Geometry check sheet. Reference: the model listing, model coordinates, mm. Face numbers are marked on the shaded views. A direction names the side the tool comes from. Give positions to 0.01 mm unless a question says otherwise; leave off trailing zeros. Write each loop counter-clockwise with the first axis right and the second up, starting at its lowest first coordinate (ties: lowest second). Pieces come first, ordered by that corner, then holes. Notation, with made-up numbers: (51, -1.75) - (90, -1.75) arc R20 ccw to (90, 24.25) - close; hole circle Ø7 at (31.5, -28.75). An arc over 180 degrees is marked (long way). Use a Markdown table: item, result.
```python
from build123d import *

# Parameters (mm, degrees)
SKETCH1_W          = 140
SKETCH1_H          = 8.92
BASE_FLANGE1_DEPTH = 2.5
EDGE_FLANGE1_DEPTH = 140
SKETCH21_R         = 1.65
CUT_EXTRUDE1_DEPTH = 78.265670645
CHAMFER1_SIZE      = 3
CHAMFER1_SIZE2     = 24.433039284
FILLET1_R          = 0.5


# Sheet-metal steps are written as plain solids
with BuildPart() as part:
    # Sketch1 → Base-Flange1 (new body)
    with BuildSketch(Plane(origin=(0, 0, 0), x_dir=(1, 0, 0), z_dir=(0, 1, 0))):
        with Locations((0, -4.46)):
            Rectangle(SKETCH1_W, SKETCH1_H)
    extrude(amount=-BASE_FLANGE1_DEPTH)

    # Edge-Flange1 section (across the edge) → Edge-Flange1 (add)
    with BuildSketch(Plane(origin=(70, -2.5, 9.759099631), x_dir=(0, -0.17364817766693427, -0.9848077530122075), z_dir=(-1, 0, 0))):
        with BuildLine():
            Line((-2.5, 0.839099631), (-2.5, 26))
            Line((-2.5, 26), (0, 26))
            Line((0, 26), (0, 0.839099631))
            ThreePointArc((0, 0.839099631), (0.233955557, 0.196312021), (0.826351822, -0.145708122))
            Line((0.826351822, -0.145708122), (0.392231378, -2.607727504))
            ThreePointArc((0.392231378, -2.607727504), (-1.681155551, -1.410657003), (-2.5, 0.839099631))
        make_face()
    extrude(amount=EDGE_FLANGE1_DEPTH)

    # Sketch21 → Cut-Extrude1 (cut, through all)
    with BuildSketch(Plane(origin=(0, 0, 0), x_dir=(1, 0, 0), z_dir=(0, 1, 0))):
        with Locations(Location((-65, -5.39, 0), (0, 0, 270))):
            Circle(SKETCH21_R)
        with Locations(Location((65, -5.39, 0), (0, 0, 270))):
            Circle(SKETCH21_R)
    extrude(amount=-CUT_EXTRUDE1_DEPTH, mode=Mode.SUBTRACT)

    # Sketch24 → Cut-Revolve2 (revolve, cut)
    with BuildSketch(Plane(origin=(65, 0, 0), x_dir=(0, 0, -1), z_dir=(1, 0, 0)), mode=Mode.PRIVATE) as cut_revolve2_sk:
        Polygon((-5.39, 0), (-5.39, -1.8), (-3.74, -1.8), (-1.94, 0), align=None)
    cut_revolve2 = revolve(cut_revolve2_sk.sketch.rotate(Axis((65, 0, 5.39), (0, 1, 0)), 180), axis=Axis((65, 0, 5.39), (0, 1, 0)), mode=Mode.SUBTRACT)

    # Mirror2: Cut-Revolve2 across plane
    add(cut_revolve2.mirror(Plane(origin=(0, 0, 0), x_dir=(0, 0, 1), z_dir=(1, 0, 0))), mode=Mode.SUBTRACT)

    # Chamfer1
    chamfer1_edges = [part.edges().sort_by_distance(p)[0] for p in [
        (70, -27.887941356, 15.504961942),
        (-70, -27.887941356, 15.504961942),
    ]]
    chamfer1_side = [part.faces().sort_by_distance(p)[0] for p in [
        (0, -27.887941356, 15.504961942),
    ]]
    chamfer(chamfer1_edges, length=CHAMFER1_SIZE, length2=CHAMFER1_SIZE2, reference=chamfer1_side[0])

    # Fillet1
    fillet1_edges = [part.edges().sort_by_distance(p)[0] for p in [
        (67, -27.887941356, 15.504961942),
        (-67, -27.887941356, 15.504961942),
        (-70, -1.25, 0),
        (70, -1.25, 0),
    ]]
    fillet(fillet1_edges, radius=FILLET1_R)


solid = part.part
```
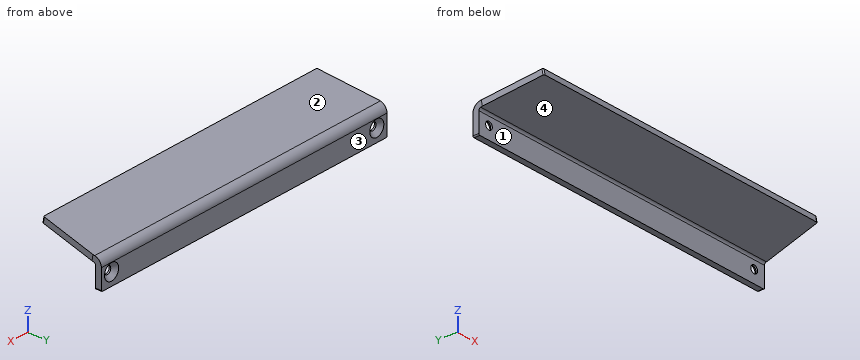
1) Section check A-A on z = 5.39. Record the boundary of the cut face in (x, y).
Working result:
| item | result |
|---|---|
| outline | (-70, -2.5) - (-66.65, -2.5) - (-66.65, -1.8) - (-68.45, 0) - (-70, 0) - close; (-63.35, -2.5) - (63.35, -2.5) - (63.35, -1.8) - (61.55, 0) - (-61.55, 0) - (-63.35, -1.8) - close; (66.65, -2.5) - (70, -2.5) - (70, 0) - (68.45, 0) - (66.65, -1.8) - close |
2) Section check D-D on y = -22.5. Record the boundary of the cut face in (x, z).
Working result:
| item | result |
|---|---|
| outline | (-67.7, 13.29) - (67.7, 13.29) - (67.64, 15.82) - (-67.64, 15.82) - close |
3) Set-up check for the marked faces 1 and 2: record each of +Z, -Z, +X, -X, +Y, -Y from which the full face is reachable in a straight line by a thin tool's end or side.
Working result:
| item | result |
|---|---|
| face 1 | -Z, +X, -X, -Y |
| face 2 | +Z, +X, -X, +Y |
4) Section check B-B on x = -65. Record the boundary of the cut face in (y, z) (3 decimals).
Working result:
| item | result |
|---|---|
| outline | (-28.105, 14.274) - (-3.326, 9.905) arc R1 cw to (-2.5, 8.92) - (-2.5, 7.04) - (-1.8, 7.04) - (0, 8.84) - (0, 8.92) arc R3.5 ccw to (-2.892, 12.367) - (-27.671, 16.736) - close; (-2.5, 0) - (0, 0) - (0, 1.94) - (-1.8, 3.74) - (-2.5, 3.74) - close |
5) Depth check by flat-ended pin: P1, Ø1, axis at x = -25, y = -6, coming from the -Z side; P2, Ø5, axis at x = -45.5, y = -14.5, coming from the -Z side; P3, Ø6, axis at y = -8, z = 14, coming from the -X side. Enter the tip coordinate at first touch or a pass-through.
Working result:
| item | result |
|---|---|
| P1 | stops at z = 10.29 |
| P2 | stops at z = 11.43 |
| P3 | stops at x = -69.79 |
6) Material ranges on L1, parallel to X at y = -1.85, z = 5.39; L2, parallel to Y at x = 33, z = 7; L3, parallel to Z at x = -65, y = -2.15, recorded low to high. Write a range as from..to.
Working result:
| item | result |
|---|---|
| L1 | x = -70..-66.65, -63.35..63.35, 66.65..70 |
| L2 | y = -2.5..0 |
| L3 | z = 0..3.74, 7.04..12.15 |
7) Section check C-C on y = -8.5. Record the boundary of the cut face in (x, z).
Working result:
| item | result |
|---|---|
| outline | (-69.44, 10.82) - (69.44, 10.82) - (69.39, 13.36) - (-69.39, 13.36) - close |
8) Mould release check, pull along Y, two halves, no side actions. Record for the marked faces 3 and 4: pulls with the +Y half, pulls with the -Y half, needs draft (parallel to the pull), parting line crosses it, or undercut.
Working result:
| item | result |
|---|---|
| face 3 | pulls with the +Y half |
| face 4 | pulls with the -Y half |
